Read the model definition and answer for the solid it produces. Units are mm, in the model's axes. Face numbers are marked on the shaded views. A direction names the side the tool comes from. Give positions to 0.01 mm unless a question says otherwise; leave off trailing zeros. Write each loop counter-clockwise with the first axis right and the second up, starting at its lowest first coordinate (ties: lowest second). Pieces come first, ordered by that corner, then holes.
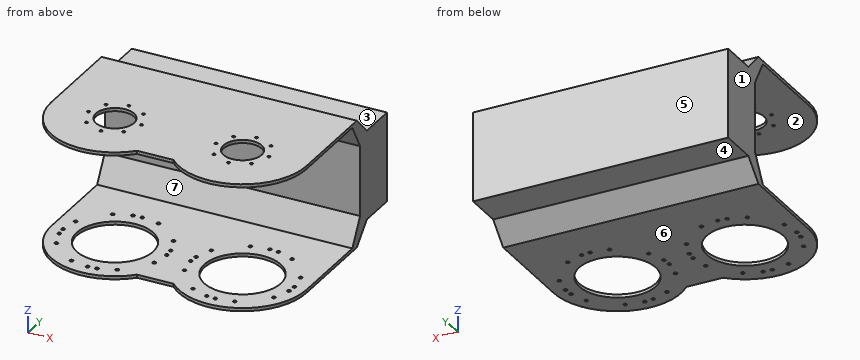
```python
from build123d import *

# Parameters (mm, degrees)
SKETCH_1_R               = 60
EXTRUDE_1_DEPTH          = 200
CUT_EXTRUDE_1_DEPTH      = 371.94473982
CUT_EXTRUDE_1_DEPTH_BACK = 371.94473982
CUT_EXTRUDE_2_DEPTH      = 371.94473982
CUT_EXTRUDE_2_DEPTH_BACK = 371.94473982
SKETCH_4_R               = 2.75
CUT_EXTRUDE_3_DEPTH      = 32.5
EXTRUDE_START            = -5
SKETCH_5_R               = 60
SKETCH_5_R_2             = 30
EXTRUDE_2_DEPTH          = 5
SKETCH_6_R               = 2.25
CUT_EXTRUDE_4_DEPTH      = 5


with BuildPart() as part:
    # 草图1 → 凸台-拉伸1 (new body)
    with BuildSketch(Plane.XY):
        with BuildLine():
            Line((200, 180), (200, 0))
            ThreePointArc((200, 0), (137.805896177, -92.578151927), (28.585715715, -70))
            Line((28.585715715, -70), (-28.585715715, -70))
            ThreePointArc((-28.585715715, -70), (-137.805896177, -92.578151927), (-200, 0))
            Line((-200, 0), (-200, 180))
            Line((-200, 180), (-200, 240))
            Line((-200, 240), (200, 240))
            Line((200, 240), (200, 180))
        make_face()
        with Locations((100, 0)):
            Circle(SKETCH_1_R, mode=Mode.SUBTRACT)
        with Locations(Location((-100, 0, 0), (0, 0, 180))):
            Circle(SKETCH_1_R, mode=Mode.SUBTRACT)
    extrude(amount=EXTRUDE_1_DEPTH)

    # 草图2 → 切除-拉伸1 (cut, two sides: drawn at the far end of the back side and taken through both)
    with BuildSketch(Plane(origin=(0, 0, 0), x_dir=(0, 0, -1), z_dir=(1, 0, 0)).offset(-CUT_EXTRUDE_1_DEPTH_BACK)):
        Polygon((-195, 136.905989232), (-195, -163.094010768), (-5, -163.094010768), (-5, 136.905989232), (-45, 160), (-155, 160), align=None)
    extrude(amount=CUT_EXTRUDE_1_DEPTH + CUT_EXTRUDE_1_DEPTH_BACK, mode=Mode.SUBTRACT)

    # 草图3 → 切除-拉伸2 (cut, two sides: drawn at the far end of the back side and taken through both)
    with BuildSketch(Plane(origin=(0, 0, 0), x_dir=(0, 0, -1), z_dir=(1, 0, 0)).offset(-CUT_EXTRUDE_2_DEPTH_BACK)):
        Polygon((-170, 240), (-170, 180), (-200, 150), (-200, 240), align=None)
        Polygon((0, 240), (-30, 240), (-30, 180), (0, 150), align=None)
    extrude(amount=CUT_EXTRUDE_2_DEPTH + CUT_EXTRUDE_2_DEPTH_BACK, mode=Mode.SUBTRACT)

    # 草图4 → 切除-拉伸3 (cut)
    with BuildSketch(Plane(origin=(0, 0, 0), x_dir=(-1, 0, 0), z_dir=(0, 0, -1))):
        with Locations((-72.051017301, 76.291656595)):
            Circle(SKETCH_4_R)
        with Locations((-100, 81.25)):
            Circle(SKETCH_4_R)
        with Locations((-113.94129927, 80.045004058)):
            Circle(SKETCH_4_R)
        with Locations((-140.625, 70.364564057)):
            Circle(SKETCH_4_R)
        with Locations((-23.708343405, -27.948982699)):
            Circle(SKETCH_4_R)
        with Locations((-18.75, 0)):
            Circle(SKETCH_4_R)
        with Locations((-19.954995942, 13.94129927)):
            Circle(SKETCH_4_R)
        with Locations((-29.635435943, 40.625)):
            Circle(SKETCH_4_R)
        with Locations((-127.948982699, -76.291656595)):
            Circle(SKETCH_4_R)
        with Locations((-100, -81.25)):
            Circle(SKETCH_4_R)
        with Locations((-86.05870073, -80.045004058)):
            Circle(SKETCH_4_R)
        with Locations((-59.375, -70.364564057)):
            Circle(SKETCH_4_R)
        with Locations((-176.291656595, 27.948982699)):
            Circle(SKETCH_4_R)
        with Locations((-181.25, 0)):
            Circle(SKETCH_4_R)
        with Locations((-180.045004058, -13.94129927)):
            Circle(SKETCH_4_R)
        with Locations((-170.364564057, -40.625)):
            Circle(SKETCH_4_R)
        with Locations(Location((170.364564057, -40.625, 0), (0, 0, 90))):
            Circle(SKETCH_4_R)
        with Locations(Location((180.045004058, -13.94129927, 0), (0, 0, 90))):
            Circle(SKETCH_4_R)
        with Locations(Location((181.25, 0, 0), (0, 0, 90))):
            Circle(SKETCH_4_R)
        with Locations(Location((176.291656595, 27.948982699, 0), (0, 0, 90))):
            Circle(SKETCH_4_R)
        with Locations(Location((59.375, -70.364564057, 0), (0, 0, 90))):
            Circle(SKETCH_4_R)
        with Locations(Location((86.05870073, -80.045004058, 0), (0, 0, 90))):
            Circle(SKETCH_4_R)
        with Locations(Location((100, -81.25, 0), (0, 0, 90))):
            Circle(SKETCH_4_R)
        with Locations(Location((127.948982699, -76.291656595, 0), (0, 0, 90))):
            Circle(SKETCH_4_R)
        with Locations(Location((29.635435943, 40.625, 0), (0, 0, 90))):
            Circle(SKETCH_4_R)
        with Locations(Location((19.954995942, 13.94129927, 0), (0, 0, 90))):
            Circle(SKETCH_4_R)
        with Locations(Location((18.75, 0, 0), (0, 0, 90))):
            Circle(SKETCH_4_R)
        with Locations(Location((23.708343405, -27.948982699, 0), (0, 0, 90))):
            Circle(SKETCH_4_R)
        with Locations(Location((140.625, 70.364564057, 0), (0, 0, 90))):
            Circle(SKETCH_4_R)
        with Locations(Location((113.94129927, 80.045004058, 0), (0, 0, 90))):
            Circle(SKETCH_4_R)
        with Locations(Location((100, 81.25, 0), (0, 0, 90))):
            Circle(SKETCH_4_R)
        with Locations(Location((72.051017301, 76.291656595, 0), (0, 0, 90))):
            Circle(SKETCH_4_R)
    extrude(amount=-CUT_EXTRUDE_3_DEPTH, mode=Mode.SUBTRACT)

    # 草图5 → 凸台-拉伸2 (add)
    # profile 1 of 2: a face of its own
    with BuildSketch(Plane.XY.offset(200).offset(EXTRUDE_START)):
        with Locations(Location((-100, 0, 0), (0, 0, 180))):
            Circle(SKETCH_5_R)
        with Locations((-100, 0)):
            Circle(SKETCH_5_R_2, mode=Mode.SUBTRACT)
    # profile 2 of 2: a face of its own
    with BuildSketch(Plane.XY.offset(200).offset(EXTRUDE_START)):
        with Locations(Location((100, 0, 0), (0, 0, 90))):
            Circle(SKETCH_5_R)
        with Locations((100, 0)):
            Circle(SKETCH_5_R_2, mode=Mode.SUBTRACT)
    extrude(amount=EXTRUDE_2_DEPTH)

    # 草图6 → 切除-拉伸4 (cut)
    with BuildSketch(Plane.XY.offset(200)):
        with Locations((100, 41.5)):
            Circle(SKETCH_6_R)
        with Locations((129.344931419, 29.344931419)):
            Circle(SKETCH_6_R)
        with Locations((141.5, 0)):
            Circle(SKETCH_6_R)
        with Locations((129.344931419, -29.344931419)):
            Circle(SKETCH_6_R)
        with Locations((100, -41.5)):
            Circle(SKETCH_6_R)
        with Locations((70.655068581, -29.344931419)):
            Circle(SKETCH_6_R)
        with Locations((58.5, 0)):
            Circle(SKETCH_6_R)
        with Locations((70.655068581, 29.344931419)):
            Circle(SKETCH_6_R)
        with Locations(Location((-70.655068581, 29.344931419, 0), (0, 0, 270))):
            Circle(SKETCH_6_R)
        with Locations(Location((-58.5, 0, 0), (0, 0, 270))):
            Circle(SKETCH_6_R)
        with Locations(Location((-70.655068581, -29.344931419, 0), (0, 0, 270))):
            Circle(SKETCH_6_R)
        with Locations(Location((-100, -41.5, 0), (0, 0, 270))):
            Circle(SKETCH_6_R)
        with Locations(Location((-129.344931419, -29.344931419, 0), (0, 0, 270))):
            Circle(SKETCH_6_R)
        with Locations(Location((-141.5, 0, 0), (0, 0, 270))):
            Circle(SKETCH_6_R)
        with Locations(Location((-129.344931419, 29.344931419, 0), (0, 0, 270))):
            Circle(SKETCH_6_R)
        with Locations(Location((-100, 41.5, 0), (0, 0, 270))):
            Circle(SKETCH_6_R)
    extrude(amount=-CUT_EXTRUDE_4_DEPTH, mode=Mode.SUBTRACT)


solid = part.part
```
Item 1: Which of the six approach directions +Z, -Z, +X, -X, +Y, -Y give full straight-line access (tool end or side, diameter ignored) to the marked faces 1, 2, 3 and 4?
Result set:
face 1: +Z, -Z, -X, +Y, -Y
face 2: +X, -X, -Y
face 3: +Z, +X, -X, +Y
face 4: -Z, +X, -X, +Y
Item 2: Find the intervals of material crossed by line 1 along Z through (x, y) = (37, 63); line 2 along Y through (x, z) = (65, 145.5); line 3 along Y through (x, z) = (100, 196.3), in increasing order.
Result set:
line 1: z = 0 to 5, 195 to 200
line 2: y = 160 to 240
line 3: y = -100 to -43.75, -39.25 to -30, 30 to 39.25, 43.75 to 153.7
Item 3: Section A-A (y = -51) is taken. Write down the section's boundary in (x, z).
Result set:
outline: (-186.02, 0) - (-131.61, 0) - (-131.61, 5) - (-186.02, 5) - close; (-186.02, 195) - (186.02, 195) - (186.02, 200) - (-186.02, 200) - close; (-68.39, 0) - (68.39, 0) - (68.39, 5) - (-68.39, 5) - close; (131.61, 0) - (186.02, 0) - (186.02, 5) - (131.61, 5) - close
Item 4: Determine the mould class of the marked faces 5, 6 and 7 for opening direction Z: pulls with the +Z half, pulls with the -Z half, needs draft (parallel to the pull), parting line crosses it, or undercut.
Result set:
face 5: needs draft
face 6: pulls with the -Z half
face 7: undercut
Item 5: Each of these flat-tipped pins is pushed along its axis until it touches: pin 1 Ø10 at (x, z) = (-130.5, 70.5) entering from -Y; pin 2 Ø4 at (x, z) = (-4.5, 2.5) entering from -Y; pin 3 Ø5 at (x, y) = (-72.05, 76.29) entering from -Z; pin 4 Ø3.5 at (x, y) = (-129.34, -29.34) entering from +Z. Where does it stop, or does it pass through?
Result set:
pin 1: stops at y = 160
pin 2: stops at y = -70
pin 3: stops at z = 195
pin 4: passes through
